```python
from build123d import *

# Parameters (mm, degrees)
SKETCH1_W                                            = 46
SKETCH1_H                                            = 31.85
BOSS_EXTRUDE1_DEPTH                                  = 20
CSK_FOR_M6_HEX_SOCKET_COUNTERSUNK_CAP_SC_D           = 2.5
CSK_FOR_M6_HEX_SOCKET_COUNTERSUNK_CAP_SC_DEPTH       = 17
CSK_FOR_M6_HEX_SOCKET_COUNTERSUNK_CAP_SC_CSINK_D     = 4
CSK_FOR_M6_HEX_SOCKET_COUNTERSUNK_CAP_SC_CSINK_ANGLE = 90
CSK_FOR_M6_HEX_SOCKET_COUNTERSUNK_CAP_SC_TIP         = 0.751075774
CUT_EXTRUDE1_DEPTH                                   = 17
SKETCH9_W                                            = 22.5
SKETCH9_H                                            = 17.5
CUT_EXTRUDE2_DEPTH                                   = 0.8
FILLET1_R                                            = 1
CHAMFER3_SIZE                                        = 5
CHAMFER3_SIZE_2                                      = 1
CHAMFER4_SIZE                                        = 5
CHAMFER4_SIZE_2                                      = 1
SKETCH15_W                                           = 1.1
SKETCH15_H                                           = 1.710862934
BOSS_EXTRUDE2_DEPTH                                  = 17
FILLET2_R                                            = 0.5
SKETCH16_R                                           = 1.225
CUT_EXTRUDE5_DEPTH                                   = 2
CUT_EXTRUDE6_DEPTH                                   = 1
SKETCH18_R                                           = 3
SKETCH18_R_2                                         = 1.225
BOSS_EXTRUDE3_DEPTH                                  = 2
SKETCH19_R                                           = 2.75
CUT_EXTRUDE7_DEPTH                                   = 51.888167829
SKETCH20_R                                           = 6.5
BOSS_EXTRUDE4_DEPTH                                  = 0.5


with BuildPart() as part:
    # Sketch1 → Boss-Extrude1 (new body)
    with BuildSketch(Plane(origin=(0, 0, 0), x_dir=(1, 0, 0), z_dir=(0, 1, 0))):
        Rectangle(SKETCH1_W, SKETCH1_H)
    extrude(amount=BOSS_EXTRUDE1_DEPTH)

    # CSK for M6 Hex Socket Countersunk Cap Screw1
    with Locations(Plane(origin=(0, 20, 0), x_dir=(1, 0, 0), z_dir=(0, 1, 0))):
        with Locations((-20.8, 13.725), (-13, -13.725), (20.8, 13.725), (20.8, -13.876947284)):
            CounterSinkHole(CSK_FOR_M6_HEX_SOCKET_COUNTERSUNK_CAP_SC_D / 2, CSK_FOR_M6_HEX_SOCKET_COUNTERSUNK_CAP_SC_CSINK_D / 2, depth=CSK_FOR_M6_HEX_SOCKET_COUNTERSUNK_CAP_SC_DEPTH, counter_sink_angle=CSK_FOR_M6_HEX_SOCKET_COUNTERSUNK_CAP_SC_CSINK_ANGLE)
            with Locations((0, 0, -(CSK_FOR_M6_HEX_SOCKET_COUNTERSUNK_CAP_SC_DEPTH + CSK_FOR_M6_HEX_SOCKET_COUNTERSUNK_CAP_SC_TIP / 2))):  # 118° drill point
                Cone(0, CSK_FOR_M6_HEX_SOCKET_COUNTERSUNK_CAP_SC_D / 2, CSK_FOR_M6_HEX_SOCKET_COUNTERSUNK_CAP_SC_TIP, mode=Mode.SUBTRACT)

    # Sketch8 → Cut-Extrude1 (cut)
    with BuildSketch(Plane(origin=(0, 20, 0), x_dir=(1, 0, 0), z_dir=(0, 1, 0))):
        with BuildLine():
            Line((-21, 0.935), (-22, 0.935))
            Line((-22, 0.935), (-22, 9.935))
            Line((-22, 9.935), (-20.8, 11.225))
            ThreePointArc((-20.8, 11.225), (-18.962882693, 12.029417504), (-18.308012841, 13.925))
            Line((-18.308012841, 13.925), (18.308012841, 13.925))
            ThreePointArc((18.308012841, 13.925), (19.142606811, 11.853356921), (21.3, 11.275510257))
            Line((21.3, 11.275510257), (22.2, 11.225))
            Line((22.2, 11.225), (22.2, -11.427457541))
            Line((22.2, -11.427457541), (21.3, -11.427457541))
            ThreePointArc((21.3, -11.427457541), (19.200322601, -11.955741356), (18.300461855, -13.925))
            Line((18.300461855, -13.925), (-10.508012841, -13.925))
            ThreePointArc((-10.508012841, -13.925), (-13, -11.225), (-15.491987159, -13.925))
            Line((-15.491987159, -13.925), (-21, -13.925))
            Line((-21, -13.925), (-21, 0.935))
        make_face()
    extrude(amount=-CUT_EXTRUDE1_DEPTH, mode=Mode.SUBTRACT)

    # Sketch9 → Cut-Extrude2 (cut)
    with BuildSketch(Plane(origin=(23, 0, 0), x_dir=(0, 0, -1), z_dir=(1, 0, 0))):
        with Locations((-0.02414151, 11.25)):
            Rectangle(SKETCH9_W, SKETCH9_H)
    extrude(amount=-CUT_EXTRUDE2_DEPTH, mode=Mode.SUBTRACT)

    # Fillet1
    fillet1_edges = [part.edges().sort_by_distance(p)[0] for p in [
        (23, 10, 15.925),
        (-23, 10, 15.925),
        (-23, 10, -15.925),
        (23, 10, -15.925),
    ]]
    fillet(fillet1_edges, radius=FILLET1_R)

    # Chamfer3
    # the kernel refuses this chamfer: 5, 1 mm, written as the material it takes off along each edge
    with BuildSketch(Plane(origin=(23, 0, 27.915660431), x_dir=(-0.9999715107910817, -0.007548351224040629, 0), z_dir=(0, 0, -1))) as chamfer3_piece_1:
        Polygon((CHAMFER3_SIZE * 0.999971510791, CHAMFER3_SIZE * 0.00754835122404), (-CHAMFER3_SIZE_2 * 0.00754835122404, CHAMFER3_SIZE_2 * 0.999971510791), (0, 0), align=None)
    extrude(amount=55.831320863, mode=Mode.SUBTRACT)

    # Chamfer4
    # the kernel refuses this chamfer: 5, 1 mm, written as the material it takes off along each edge
    with BuildSketch(Plane(origin=(30.990660431, 0, -15.925), x_dir=(0, -0.007548351224040629, 0.9999715107910817), z_dir=(-1, 0, 0))) as chamfer4_piece_1:
        Polygon((CHAMFER4_SIZE * 0.999971510791, CHAMFER4_SIZE * 0.00754835122404), (-CHAMFER4_SIZE_2 * 0.00754835122404, CHAMFER4_SIZE_2 * 0.999971510791), (0, 0), align=None)
    extrude(amount=65.981320863, mode=Mode.SUBTRACT)
    with BuildSketch(Plane(origin=(-34.990660431, 0, 15.925), x_dir=(0, 0.9826554028509425, 0.18544098588999117), z_dir=(1, 0, 0))) as chamfer4_piece_2:
        Polygon((CHAMFER4_SIZE_2 * 0.982655402851, -CHAMFER4_SIZE_2 * 0.18544098589), (-CHAMFER4_SIZE * 0.18544098589, -CHAMFER4_SIZE * 0.982655402851), (0, 0), align=None)
    extrude(amount=65.981320863, mode=Mode.SUBTRACT)

    # Sketch15 → Boss-Extrude2 (add)
    with BuildSketch(Plane(origin=(0, 3, 0), x_dir=(1, 0, 0), z_dir=(0, 1, 0))):
        with Locations((21.65, 10.855431467)):
            Rectangle(SKETCH15_W, SKETCH15_H)
        with Locations((21.65, -10.855431467)):
            Rectangle(SKETCH15_W, SKETCH15_H)
    extrude(amount=BOSS_EXTRUDE2_DEPTH)

    # Fillet2
    fillet2_edges = [part.edges().sort_by_distance(p)[0] for p in [
        (21.65, 3, -10),
        (21.65, 3, 10),
        (22.6, 2.5, 11.27414151),
        (22.6, 2.5, -11.22585849),
    ]]
    fillet(fillet2_edges, radius=FILLET2_R)

    # Sketch16 → Cut-Extrude5 (cut)
    with BuildSketch(Plane(origin=(0, 3, 0), x_dir=(1, 0, 0), z_dir=(0, 1, 0))):
        with Locations(Location((-15, 5.435, 0), (0, 0, 270))):
            Circle(SKETCH16_R)
        with Locations(Location((-5, 5, 0), (0, 0, 270))):
            Circle(SKETCH16_R)
        with Locations(Location((-5, -5, 0), (0, 0, 90))):
            Circle(SKETCH16_R)
    extrude(amount=-CUT_EXTRUDE5_DEPTH, mode=Mode.SUBTRACT)

    # Sketch17 → Cut-Extrude6 (cut)
    with BuildSketch(Plane(origin=(0, 3, 0), x_dir=(1, 0, 0), z_dir=(0, 1, 0))):
        with BuildLine():
            Line((-22, 0.935), (-22, 9.935))
            Line((-22, 9.935), (-15, 9.935))
            ThreePointArc((-15, 9.935), (-10.5, 5.435), (-15, 0.935))
            Line((-15, 0.935), (-22, 0.935))
        make_face()
    extrude(amount=-CUT_EXTRUDE6_DEPTH, mode=Mode.SUBTRACT)

    # Sketch18 → Boss-Extrude3 (add)
    with BuildSketch(Plane(origin=(0, 3, 0), x_dir=(1, 0, 0), z_dir=(0, 1, 0))):
        with Locations(Location((7.81, 0, 0), (0, 0, 270))):
            Circle(SKETCH18_R)
        with Locations(Location((7.81, 0, 0), (0, 0, 270))):
            Circle(SKETCH18_R_2, mode=Mode.SUBTRACT)
    extrude(amount=BOSS_EXTRUDE3_DEPTH)

    # Sketch19 → Cut-Extrude7 (cut, through all)
    with BuildSketch(Plane(origin=(-21, 0, 0), x_dir=(0, 0, -1), z_dir=(1, 0, 0))):
        with Locations((-2.925, 9)):
            Circle(SKETCH19_R)
    extrude(amount=-CUT_EXTRUDE7_DEPTH, mode=Mode.SUBTRACT)

    # Sketch20 → Boss-Extrude4 (add)
    with BuildSketch(Plane.XZ):
        with Locations(Location((7.81, 0, 0), (0, 0, 270))):
            Circle(SKETCH20_R)
    extrude(amount=BOSS_EXTRUDE4_DEPTH)


solid = part.part
```
Verification items for the finished model (mm, model axes). A direction names the side the tool comes from. Coordinates: 2 decimals unless noted, no trailing zeros. Write each loop counter-clockwise with the first axis right and the second up, starting at its lowest first coordinate (ties: lowest second). Pieces come first, ordered by that corner, then holes. Notation, with made-up numbers: M -29,-21 L 0,-21 A15 ccw 0,6 Z; hole C -37.5,-31 d9. An arc over 180 degrees is marked long. One line per item, written item: value.
Item 1: Access from +Z, -Z, +X, -X, +Y, -Y to the whole of each face (thin tool, end or side, straight path). Record for faces 1 (the cylindrical face through (19.61, 11.01, 13.5)), 2 (the cylindrical face through (-21.99, 11.32, 1.45)), 3 (the flat face through (22, 12, 10)).
Check sheet entries:
face 1: +Y
face 2: +X, -X
face 3: +X, +Y
Item 2: Section check C-C, the plane y = 18. State how many separate pieces and enclosed holes the cut face has, plus the area to 3 significant figures.
Check sheet entries:
separate pieces: 1
enclosed holes: 4
area: 251 mm^2
Item 3: Mould release check, pull along Z, two halves, no side actions. Record for faces 4 (the cylindrical face through (22.7, 10.6, 15.64)), 5 (the cylindrical face through (-12.942, 11.619, 11.226)), 6 (the flat face through (22, 12, -10)), 7 (the flat face through (-3, 0, 0)): pulls with the +Z half, pulls with the -Z half, needs draft (parallel to the pull), parting line crosses it, or undercut.
Check sheet entries:
face 4: pulls with the +Z half
face 5: undercut
face 6: undercut
face 7: needs draft
Item 4: Section check D-D, the plane z = -5. Record the boundary of the cut face in (x, y) (3 decimals).
Check sheet entries:
outline: M -23,0 L 3.657,0 L 3.657,-0.5 L 11.963,-0.5 L 11.963,0 L 18,0 L 23,1 L 23,2.5 L 22.2,2.5 L 22.2,3 L -3.775,3 L -3.775,1 L -6.225,1 L -6.225,3 L -10.521,3 L -10.521,2 L -13.855,2 L -13.855,1 L -16.145,1 L -16.145,2 L -22,2 L -22,20 L -23,20 Z
Item 5: Section check A-A, the plane x = 7.81. Record the boundary of the cut face in (y, z) (3 decimals), plus the area to 3 significant figures.
Check sheet entries:
outline: M -0.5,-6.5 L 0,-6.5 L 0,-10.925 L 1,-15.925 L 20,-15.925 L 20,-13.925 L 3,-13.925 L 3,-3 L 5,-3 L 5,-1.225 L 3,-1.225 L 3,1.225 L 5,1.225 L 5,3 L 3,3 L 3,13.925 L 20,13.925 L 20,15.925 L 1,15.925 L 0,10.925 L 0,6.5 L -0.5,6.5 Z
area: 172 mm^2
Item 6: Gauge pin test, flat ends, axial feed: pin 1 Ø0.7 at (x, z) = (-5.5, -4.5) entering from +Y; pin 2 Ø5 at (x, z) = (-8, 4) entering from -Y; pin 3 Ø4 at (x, z) = (-13, 13.725) entering from -Y. Record the tip position at first contact, or that the pin passes through.
Check sheet entries:
pin 1: stops at y = 1
pin 2: stops at y = 0
pin 3: stops at y = 0.16
Item 7: Section check B-B, the plane z = 5. Record the boundary of the cut face in (x, y) (3 decimals).
Check sheet entries:
outline: M -23,0 L 3.657,0 L 3.657,-0.5 L 11.963,-0.5 L 11.963,0 L 18,0 L 23,1 L 23,2.5 L 22.2,2.5 L 22.2,3 L -3.775,3 L -3.775,1 L -6.225,1 L -6.225,3 L -21,3 L -21,7.195 L -23,7.195 Z; M -23,10.805 L -21,10.805 L -21,20 L -23,20 Z
Item 8: Scan lines: line 1 along Z through (x, y) = (20.8, 14.75) (3 decimals); line 2 along Z through (x, y) = (-13, 16.25) (3 decimals); line 3 along Z through (x, y) = (15.5, 8.5) (3 decimals). Record each from-to range of solid material in increasing order.
Check sheet entries:
line 1: z = -15.925 to -14.975, -12.475 to -11.225, 11.377 to 12.627, 15.127 to 15.925
line 2: z = -15.925 to -13.925, 11.225 to 12.475, 14.975 to 15.925
line 3: z = -15.925 to -13.925, 13.925 to 15.925
